from build123d import *

# Parameters (mm, degrees)
CELL_BLOCK_SKETCH_W  = 127.601132068
CELL_BLOCK_SKETCH_H  = 227.325
BOSS_EXTRUDE1_DEPTH  = 5
CELL_HOLES_PATTERN_R = 10.875
CUT_EXTRUDE1_DEPTH   = 5
SKETCH1_R            = 10.875
CUT_EXTRUDE2_DEPTH   = 5
SKETCH3_W            = 16
SKETCH3_H            = 227.325
BOSS_EXTRUDE3_DEPTH  = 5
SKETCH4_R            = 3.25
CUT_EXTRUDE3_DEPTH   = 5


with BuildPart() as part:
    # Cell Block Sketch → Boss-Extrude1 (new body)
    with BuildSketch(Plane(origin=(0, 0, 0), x_dir=(1, 0, 0), z_dir=(0, 1, 0))):
        Rectangle(CELL_BLOCK_SKETCH_W, CELL_BLOCK_SKETCH_H)
    extrude(amount=BOSS_EXTRUDE1_DEPTH)

    # Cell Holes Pattern → Cut-Extrude1 (cut)
    with BuildSketch(Plane(origin=(0, 0, 0), x_dir=(1, 0, 0), z_dir=(0, 1, 0))):
        with Locations(Location((-33.150283017, 86.4125, 0), (0, 0, 270))):
            Circle(CELL_HOLES_PATTERN_R)
        with Locations((-53.025566034, 97.8875)):
            Circle(CELL_HOLES_PATTERN_R)
        with Locations(Location((-13.275, 97.8875, 0), (0, 0, 270))):
            Circle(CELL_HOLES_PATTERN_R)
        with Locations((-53.025566034, 74.9375)):
            Circle(CELL_HOLES_PATTERN_R)
        with Locations(Location((-33.150283017, 63.4625, 0), (0, 0, 270))):
            Circle(CELL_HOLES_PATTERN_R)
        with Locations(Location((-13.275, 74.9375, 0), (0, 0, 270))):
            Circle(CELL_HOLES_PATTERN_R)
        with Locations((-53.025566034, 51.9875)):
            Circle(CELL_HOLES_PATTERN_R)
        with Locations(Location((-33.150283017, 40.5125, 0), (0, 0, 270))):
            Circle(CELL_HOLES_PATTERN_R)
        with Locations(Location((-13.275, 51.9875, 0), (0, 0, 270))):
            Circle(CELL_HOLES_PATTERN_R)
        with Locations((-53.025566034, 29.0375)):
            Circle(CELL_HOLES_PATTERN_R)
        with Locations(Location((-33.150283017, 17.5625, 0), (0, 0, 270))):
            Circle(CELL_HOLES_PATTERN_R)
        with Locations(Location((-13.275, 29.0375, 0), (0, 0, 270))):
            Circle(CELL_HOLES_PATTERN_R)
        with Locations((-53.025566034, 6.0875)):
            Circle(CELL_HOLES_PATTERN_R)
        with Locations(Location((-33.150283017, -5.3875, 0), (0, 0, 270))):
            Circle(CELL_HOLES_PATTERN_R)
        with Locations(Location((-13.275, 6.0875, 0), (0, 0, 270))):
            Circle(CELL_HOLES_PATTERN_R)
        with Locations((-53.025566034, -16.8625)):
            Circle(CELL_HOLES_PATTERN_R)
        with Locations(Location((-33.150283017, -28.3375, 0), (0, 0, 270))):
            Circle(CELL_HOLES_PATTERN_R)
        with Locations(Location((-13.275, -16.8625, 0), (0, 0, 270))):
            Circle(CELL_HOLES_PATTERN_R)
        with Locations((-53.025566034, -39.8125)):
            Circle(CELL_HOLES_PATTERN_R)
        with Locations(Location((-33.150283017, -51.2875, 0), (0, 0, 270))):
            Circle(CELL_HOLES_PATTERN_R)
        with Locations(Location((-13.275, -39.8125, 0), (0, 0, 270))):
            Circle(CELL_HOLES_PATTERN_R)
        with Locations((-53.025566034, -62.7625)):
            Circle(CELL_HOLES_PATTERN_R)
        with Locations(Location((-33.150283017, -74.2375, 0), (0, 0, 270))):
            Circle(CELL_HOLES_PATTERN_R)
        with Locations(Location((-13.275, -62.7625, 0), (0, 0, 270))):
            Circle(CELL_HOLES_PATTERN_R)
        with Locations((-53.025566034, -85.7125)):
            Circle(CELL_HOLES_PATTERN_R)
        with Locations(Location((-33.150283017, -97.1875, 0), (0, 0, 270))):
            Circle(CELL_HOLES_PATTERN_R)
        with Locations(Location((-13.275, -85.7125, 0), (0, 0, 270))):
            Circle(CELL_HOLES_PATTERN_R)
    extrude(amount=CUT_EXTRUDE1_DEPTH, mode=Mode.SUBTRACT)

    # Sketch1 → Cut-Extrude2 (cut)
    with BuildSketch(Plane(origin=(0, 5, 0), x_dir=(1, 0, 0), z_dir=(0, 1, 0))):
        with Locations(Location((13.275, 86.4125, 0), (0, 0, 270))):
            Circle(SKETCH1_R)
        with Locations(Location((33.150283017, 97.8875, 0), (0, 0, 270))):
            Circle(SKETCH1_R)
        with Locations((53.025566034, 86.4125)):
            Circle(SKETCH1_R)
        with Locations(Location((13.275, 63.4625, 0), (0, 0, 270))):
            Circle(SKETCH1_R)
        with Locations(Location((33.150283017, 74.9375, 0), (0, 0, 270))):
            Circle(SKETCH1_R)
        with Locations((53.025566034, 63.4625)):
            Circle(SKETCH1_R)
        with Locations(Location((13.275, 40.5125, 0), (0, 0, 270))):
            Circle(SKETCH1_R)
        with Locations(Location((33.150283017, 51.9875, 0), (0, 0, 270))):
            Circle(SKETCH1_R)
        with Locations((53.025566034, 40.5125)):
            Circle(SKETCH1_R)
        with Locations(Location((13.275, 17.5625, 0), (0, 0, 270))):
            Circle(SKETCH1_R)
        with Locations(Location((33.150283017, 29.0375, 0), (0, 0, 270))):
            Circle(SKETCH1_R)
        with Locations((53.025566034, 17.5625)):
            Circle(SKETCH1_R)
        with Locations(Location((13.275, -5.3875, 0), (0, 0, 270))):
            Circle(SKETCH1_R)
        with Locations(Location((33.150283017, 6.0875, 0), (0, 0, 270))):
            Circle(SKETCH1_R)
        with Locations((53.025566034, -5.3875)):
            Circle(SKETCH1_R)
        with Locations(Location((13.275, -28.3375, 0), (0, 0, 270))):
            Circle(SKETCH1_R)
        with Locations(Location((33.150283017, -16.8625, 0), (0, 0, 270))):
            Circle(SKETCH1_R)
        with Locations((53.025566034, -28.3375)):
            Circle(SKETCH1_R)
        with Locations(Location((13.275, -51.2875, 0), (0, 0, 270))):
            Circle(SKETCH1_R)
        with Locations(Location((33.150283017, -39.8125, 0), (0, 0, 270))):
            Circle(SKETCH1_R)
        with Locations((53.025566034, -51.2875)):
            Circle(SKETCH1_R)
        with Locations(Location((13.275, -74.2375, 0), (0, 0, 270))):
            Circle(SKETCH1_R)
        with Locations(Location((33.150283017, -62.7625, 0), (0, 0, 270))):
            Circle(SKETCH1_R)
        with Locations((53.025566034, -74.2375)):
            Circle(SKETCH1_R)
        with Locations(Location((13.275, -97.1875, 0), (0, 0, 270))):
            Circle(SKETCH1_R)
        with Locations(Location((33.150283017, -85.7125, 0), (0, 0, 270))):
            Circle(SKETCH1_R)
        with Locations((53.025566034, -97.1875)):
            Circle(SKETCH1_R)
    extrude(amount=-CUT_EXTRUDE2_DEPTH, mode=Mode.SUBTRACT)

    # Sketch3 → Boss-Extrude3 (add)
    with BuildSketch(Plane(origin=(0, 0, 0), x_dir=(1, 0, 0), z_dir=(0, 1, 0))):
        with Locations((-71.800566034, 0)):
            Rectangle(SKETCH3_W, SKETCH3_H)
    boss_extrude3 = extrude(amount=BOSS_EXTRUDE3_DEPTH)

    # Mirror1: Boss-Extrude3 across plane
    add(boss_extrude3.mirror(Plane(origin=(0, 0, 0), x_dir=(0, 0, 1), z_dir=(1, 0, 0))))

    # Sketch4 → Cut-Extrude3 (cut)
    with BuildSketch(Plane(origin=(0, 5, 0), x_dir=(1, 0, 0), z_dir=(0, 1, 0))):
        with Locations(Location((-71.800566034, 0, 0), (0, 0, 270))):
            Circle(SKETCH4_R)
        with Locations(Location((-71.800566034, -42, 0), (0, 0, 270))):
            Circle(SKETCH4_R)
        with Locations(Location((-71.800566034, -84, 0), (0, 0, 270))):
            Circle(SKETCH4_R)
        with Locations(Location((-71.800566034, 42, 0), (0, 0, 270))):
            Circle(SKETCH4_R)
        with Locations(Location((-71.800566034, 84, 0), (0, 0, 270))):
            Circle(SKETCH4_R)
    cut_extrude3 = extrude(amount=-CUT_EXTRUDE3_DEPTH, mode=Mode.SUBTRACT)

    # Mirror2: Cut-Extrude3 across plane
    add(cut_extrude3.mirror(Plane(origin=(0, 0, 0), x_dir=(0, 0, 1), z_dir=(1, 0, 0))), mode=Mode.SUBTRACT)


solid = part.part
The listing builds one solid part. Answer for the finished solid, in the listing's coordinates (mm). Give positions to 0.01 mm unless a question says otherwise; leave off trailing zeros. Loops run counter-clockwise (first coordinate to the right, second up) from the corner with the lowest first, then second, coordinate; pieces in that order, holes last. Notation, with made-up numbers: (84.5, 70.5) - (94.5, 70.5) arc R21 cw to (94.5, 104.5) - close; hole circle Ø6 at (10.5, 2). An arc over 180 degrees is marked (long way). Answer as a JSON object with one key per item and string values.
1. A cutting plane is placed at A-A (z = -57.5). Write down the section's boundary in (x, y), then the cut area to 3 significant figures.
Determined:
{"outline": "(-79.8, 0) - (-62.4, 0) - (-62.4, 5) - (-79.8, 5) - close; (-43.65, 0) - (-42.25, 0) - (-42.25, 5) - (-43.65, 5) - close; (-24.06, 0) - (-22.65, 0) - (-22.65, 5) - (-24.06, 5) - close; (-3.9, 0) - (4.18, 0) - (4.18, 5) - (-3.9, 5) - close; (22.37, 0) - (23.78, 0) - (23.78, 5) - (22.37, 5) - close; (42.52, 0) - (43.93, 0) - (43.93, 5) - (42.52, 5) - close; (62.12, 0) - (79.8, 0) - (79.8, 5) - (62.12, 5) - close", "area": "244 mm²"}
2. Find the intervals of material crossed by L1, parallel to X at y = 0.5, z = -6; L2, parallel to X at y = 4.6, z = -102.5, in increasing order. Write a range as [from, to].
Determined:
{"L1": "[-79.8, -63.8], [-42.15, -24.15], [-2.4, 22.28], [44.02, 79.8]", "L2": "[-79.8, -62.87], [-43.18, -23.12], [-3.43, 23.3], [43, 79.8]"}
3. A cutting plane is placed at B-B (x = -58.5). Give the number of separate pieces and of enclosed holes in the cut face, then the cut area to 3 significant figures.
Determined:
{"separate pieces": "10", "enclosed holes": "0", "area": "291 mm²"}
4. For a pull along X with two mould halves and no side action, classify faces 1 (the cylindrical face through (42.16, 2.54, 27.88)), 2 (the cylindrical face through (33.63, 2.54, -85.8)) as pulls with the +X half, pulls with the -X half, needs draft (parallel to the pull), parting line crosses it, or undercut.
Determined:
{"face 1": "undercut", "face 2": "undercut"}
5. A cutting plane is placed at C-C (z = -10.5). Write down the section's boundary in (x, y), then the cut area to 3 significant figures.
Determined:
{"outline": "(-79.8, 0) - (-62.97, 0) - (-62.97, 5) - (-79.8, 5) - close; (-43.09, 0) - (-41.42, 0) - (-41.42, 5) - (-43.09, 5) - close; (-24.88, 0) - (-23.21, 0) - (-23.21, 5) - (-24.88, 5) - close; (-3.34, 0) - (5.01, 0) - (5.01, 5) - (-3.34, 5) - close; (21.54, 0) - (23.21, 0) - (23.21, 5) - (21.54, 5) - close; (43.09, 0) - (44.76, 0) - (44.76, 5) - (43.09, 5) - close; (61.3, 0) - (79.8, 0) - (79.8, 5) - (61.3, 5) - close", "area": "252 mm²"}
